For this review, take the finished solid that the model builds, in its own axes (mm). A direction names the side the tool comes from. Coordinates: 2 decimals unless noted, no trailing zeros. Order: outer loops, then holes, each group sorted by start corner. A loop starts at its lowest first (then second) coordinate and runs counter-clockwise, first axis right, second up. Notation, with made-up numbers: (39.25, -26.75) -> (83.25, -26.75) arc R23 ccw to (83.25, 5.25) -> close; hole circle Ø10 at (71, -30.5). An arc over 180 degrees is marked (long way). Answer as a JSON object with one key per item and string values. Group by question number.
1) For pin 1 (1 mm diameter, centred on x = -477, y = -4, fed in from -Z); pin 2 (5 mm diameter, centred on x = -285, y = 7.5, fed in from +Z); pin 3 (8 mm diameter, centred on x = -144.5, y = -4, fed in from +Z), all flat-tipped, find the tip position at first contact; note any pin that passes through.
2) Add section B-B, the plane z = 125. Write out the cut boundary in (x, y), then the cut area to 3 significant figures.
3) Wall thickness on L1, parallel to Z at x = -492, y = -5; L2, parallel to X at y = -6.5, z = -201.5; L3, parallel to X at y = 9, z = -209.5: over which ranges is each line inside the solid? List them lowest first.
4) Add section C-C, the plane x = -24.5. Write out the cut boundary in (y, z).
5) Machinability: for faces 1 (the flat face through (25, 0, 0)), 2 (the flat face through (-560, 0, 109)), which of the approach directions +Z, -Z, +X, -X, +Y, -Y give a long, thin tool a straight path to every point of the face, cutting with its end or side? Answer none if there is none.
6) Add section A-A, the plane y = 5.75. Write out the cut boundary in (x, z).
Solid Edge part; units mm, degrees
sketch "Sketch1" plane through (0, 0, 0) normal (0, -1, 0) x (1, 0, 0)
  line L0 (50, -342.5) -> (50, 0)
  line L1 (0, 0) -> (50, 0)
  line L2 (-560, 160) -> (0, 0)
  line L3 (-560, 60) -> (-560, 160)
  line L4 (-50, -342.5) -> (-560, 60)
  line L5 (50, -342.5) -> (-50, -342.5)
extrude "Protrusion1" add sketch "Sketch1" along normal mid plane 20
Output values:
{
 "1": {"pin 1": "stops at z = -5.9", "pin 2": "stops at z = 82.14", "pin 3": "stops at z = 42.43"},
 "2": {"outline": "(-560, -10) -> (-437.5, -10) -> (-437.5, 10) -> (-560, 10) -> close", "area": "2,450 mm²"},
 "3": {"L1": "z = 6.33 to 140.57", "L2": "x = -228.66 to 50", "L3": "x = -218.52 to 50"},
 "4": {"outline": "(-10, -342.5) -> (10, -342.5) -> (10, 7) -> (-10, 7) -> close"},
 "5": {"face 1": "+Z, +X, +Y, -Y", "face 2": "+Z, -Z, -X, +Y, -Y"},
 "6": {"outline": "(-560, 60) -> (-50, -342.5) -> (50, -342.5) -> (50, 0) -> (0, 0) -> (-560, 160) -> close"}
}
